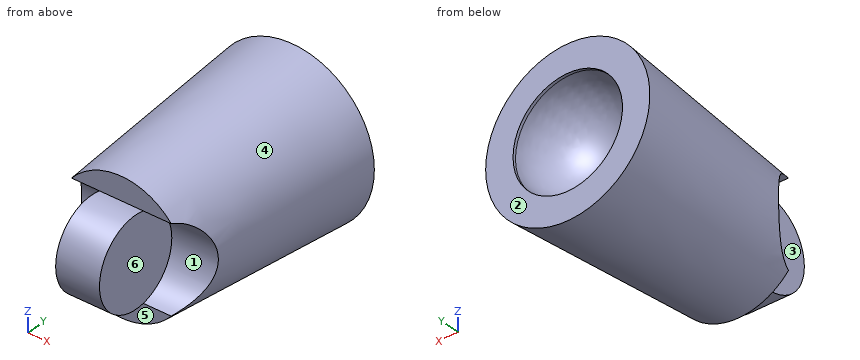
```python
from build123d import *

# Parameters (mm, degrees)
F2_R     = 5.08
F3_DEPTH = 25.4
F4_DEPTH = 2.54


with BuildPart() as f1:
    # F0 (on Top) → F1 (revolve)
    with BuildSketch(Plane.XY):
        with BuildLine():
            ThreePointArc((6.34011, 10.678397), (6.347527, 10.501329), (6.35, 10.324123))
            ThreePointArc((6.35, 10.324123), (4.490128, 5.833995), (0, 3.974123))
            Line((0, 3.974123), (0, -13.321603))
            Line((0, -13.321603), (7.62, -13.321603))
            Line((7.62, -13.321603), (9.51511, 10.678397))
            Line((9.51511, 10.678397), (6.34011, 10.678397))
        make_face()
    revolve(axis=Axis((0, -4.67374, 0), (0, 1, 0)))

    # F2 (on Right) → F3 (cut, symmetric)
    with BuildSketch(Plane.YZ):
        with Locations((-14.397663, 0)):
            Circle(F2_R)
    extrude(amount=F3_DEPTH, both=True, mode=Mode.SUBTRACT)

    # F2 (on Right) → F4 (join, symmetric)
    with BuildSketch(Plane.YZ):
        with Locations((-14.397663, 0)):
            Circle(F2_R)
    extrude(amount=F4_DEPTH, both=True)


solid = f1.part
```
The listing builds one solid part. Answer for the finished solid, in the listing's coordinates (mm). Face numbers are marked on the shaded views. A direction names the side the tool comes from. Round coordinates to 2 decimals unless told otherwise and drop trailing zeros. Order: outer loops, then holes, each group sorted by start corner. A loop starts at its lowest first (then second) coordinate and runs counter-clockwise, first axis right, second up. Notation, with made-up numbers: (-26, -23.5) - (17, -23.5) arc R23 cw to (17, 12.5) - close; hole circle Ø2 at (38.25, -34). An arc over 180 degrees is marked (long way). Put each result on its own line as item: value. Start each with the question number.
(1) Find section A-A (y = -12.5). Give the vertices of the cut face in (x, z), plus the area to 3 significant figures.
(2) Straight lines are drawn through the part: probe 1 along Z at (x, y) = (-6.75, 7.5); probe 2 along Z at (x, y) = (3.25, 6); probe 3 along Z at (x, y) = (0.75, -15). For each, find the intervals that lie inside material, in ascending order. Write a range as from..to.
(3) Find section D-D (y = 1). Give the vertices of the cut face in (x, z).
(4) Find section C-C (y = -17.5). Give the vertices of the cut face in (x, z).
(5) Determine the mould class of the marked faces 4, 5 and 6 for opening direction Z: released by +Z, released by -Z, zero draft, split by the parting line, or undercut.
(6) Find section B-B (y = -4.5). Give the vertices of the cut face in (x, z).
(7) For the marked faces 1, 2 and 3, determine the directions among +Z, -Z, +X, -X, +Y, -Y from which every point of the face is accessible in a straight line to the end or side of a thin tool.
(8) Given P1, Ø6, axis at x = -7, z = 4.5, coming from the -Y side; P2, Ø6, axis at y = 3.5, z = -7.5, coming from the -X side; P3, Ø8, axis at x = 7, y = -9, coming from the +Z side, each flat-ended and moving along its own axis, determine where each tip first touches the part or whether it passes through.
Reply:
1. outline: (-6.07, -4.71) arc R7.68 ccw to (6.07, -4.71) - (2.54, -4.71) - (2.54, 4.71) - (6.07, 4.71) arc R7.68 ccw to (-6.07, 4.71) - (-2.54, 4.71) - (-2.54, -4.71) - close
1. area: 98.2 mm^2
2. probe 1: -6.35..6.35
2. probe 2: -8.55..-3.33, 3.33..8.55
2. probe 3: -5.04..5.04
3. outline: circle Ø17.5 at (0, 0)
4. outline: (-2.54, -4.02) - (2.54, -4.02) - (2.54, 4.02) - (-2.54, 4.02) - close
5. face 4: split by the parting line
5. face 5: zero draft
5. face 6: undercut
6. outline: circle Ø16.63 at (0, 0)
7. face 1: +X, -Y
7. face 2: +Z, -Z, +X, -X, +Y
7. face 3: -X, -Y
8. P1: y = -13.32
8. P2: x = -7.76
8. P3: z = 7.41
